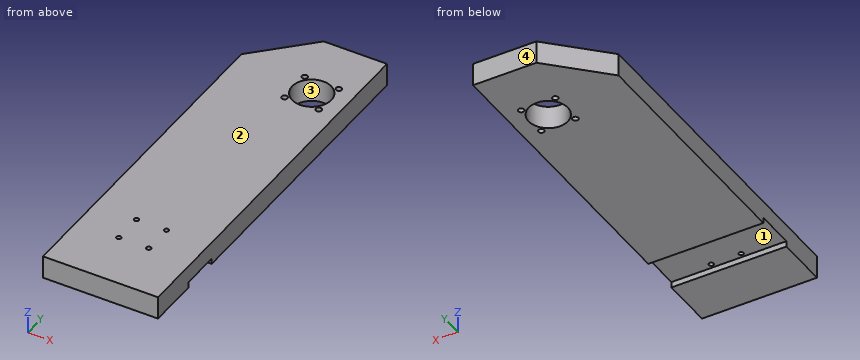
from build123d import *

# Parameters (mm, degrees)
SKETCH1_W           = 100
SKETCH1_H           = 337
SKETCH1_R           = 17
SKETCH1_R_2         = 2.5
SKETCH1_R_3         = 2
BOSS_EXTRUDE1_DEPTH = 20
CHAMFER1_SIZE       = 45
SKETCH2_W           = 100
SKETCH2_H           = 34
CUT_EXTRUDE1_DEPTH  = 5


with BuildPart() as part:
    # Sketch1 → Boss-Extrude1 (new body)
    with BuildSketch(Plane.XY):
        with Locations((47.704546062, 452.000370419)):
            Rectangle(SKETCH1_W, SKETCH1_H)
        with Locations((67.704546062, 560.500370419)):
            Circle(SKETCH1_R, mode=Mode.SUBTRACT)
        with Locations((82.553788467, 575.349612824)):
            Circle(SKETCH1_R_2, mode=Mode.SUBTRACT)
        with Locations((82.553788467, 545.651128014)):
            Circle(SKETCH1_R_2, mode=Mode.SUBTRACT)
        with Locations((52.855303657, 545.651128014)):
            Circle(SKETCH1_R_2, mode=Mode.SUBTRACT)
        with Locations((52.855303657, 575.349612824)):
            Circle(SKETCH1_R_2, mode=Mode.SUBTRACT)
        with Locations((34.704546062, 358.500370419)):
            Circle(SKETCH1_R_3, mode=Mode.SUBTRACT)
        with Locations(Location((60.704546062, 358.500370419, 0), (0, 0, 180))):
            Circle(SKETCH1_R_3, mode=Mode.SUBTRACT)
        with Locations((60.704546062, 332.500370419)):
            Circle(SKETCH1_R_3, mode=Mode.SUBTRACT)
        with Locations(Location((34.704546062, 332.500370419, 0), (0, 0, 180))):
            Circle(SKETCH1_R_3, mode=Mode.SUBTRACT)
    extrude(amount=BOSS_EXTRUDE1_DEPTH)

    # Chamfer1
    chamfer1_edges = [part.edges().sort_by_distance(p)[0] for p in [
        (-2.295453938, 620.500370419, 10),
    ]]
    chamfer(chamfer1_edges, length=CHAMFER1_SIZE)

    # Sketch2 → Cut-Extrude1 (cut)
    with BuildSketch(Plane.XY):
        with Locations((47.704546062, 345.500370419)):
            Rectangle(SKETCH2_W, SKETCH2_H)
    extrude(amount=CUT_EXTRUDE1_DEPTH, mode=Mode.SUBTRACT)


solid = part.part
The model under review builds one solid part; all positions refer to its coordinate system, in mm. Face numbers are marked on the shaded views. Round coordinates to 2 decimals unless told otherwise and drop trailing zeros. Write each loop counter-clockwise with the first axis right and the second up, starting at its lowest first coordinate (ties: lowest second). Pieces come first, ordered by that corner, then holes. Notation, with made-up numbers: M 65.25,-28 L 99.25,-28 A12 ccw 99.25,-14 Z; hole C -1.75,-36 d6. An arc over 180 degrees is marked long. Answer as CSV lines item,"result". Start each with the question number.
Q1. Consider section C-C, the plane y = 593. Give the boundary of the cut face in (x, z), then the cut area to 3 significant figures.
Q2. The part is to be moulded in two halves that separate along Y. For the marked faces 1, 2, 3 and 4, say which applies: +Y half, -Y half, draft (parallel to the pull), parting line (faces both ways), or undercut.
Q3. Clearance check with flat-ended pins moving along their axes: P1, Ø5, axis at x = 34.7, y = 358.5, coming from the -Z side; P2, Ø1, axis at x = 17.5, z = 12.5, coming from the +Y side; P3, Ø1.5, axis at x = 24, z = 2, coming from the +Y side. State where each tip first meets the part, or that it passes through.
Q4. Consider section A-A, the plane z = 11.5. State how many separate pieces and enclosed holes the cut face has, then the cut area to 3 significant figures.
Q5. Wall thickness on line 1 along X through (y, z) = (574, 3.75); line 2 along Y through (x, z) = (59.5, 4.5); line 3 along Y through (x, z) = (68, 14): over which ranges is each line inside the solid? List them lowest first.
Q6. Consider section B-B, the plane x = 12.5. Give the boundary of the cut face in (y, z).
Result set:
1,outline,"M 15.2,0 L 97.7,0 L 97.7,20 L 15.2,20 Z"
1,area,"1,650 mm²"
2,face 1,"undercut"
2,face 2,"draft"
2,face 3,"undercut"
2,face 4,"+Y half"
3,P1,"stops at z = 5"
3,P2,"stops at y = 595.8"
3,P3,"stops at y = 602.55"
4,separate pieces,"1"
4,enclosed holes,"9"
4,area,"31,700 mm²"
5,line 1,"x = -2.3 to 50.75, 54.96 to 57.37, 78.04 to 80.45, 84.66 to 97.7"
5,line 2,"y = 283.5 to 328.5, 362.5 to 545.61, 575.39 to 620.5"
5,line 3,"y = 283.5 to 543.5, 577.5 to 620.5"
6,outline,"M 283.5,0 L 328.5,0 L 328.5,5 L 362.5,5 L 362.5,0 L 590.3,0 L 590.3,20 L 283.5,20 Z"
